from build123d import *

# Parameters (mm, degrees)
SKETCH1_R           = 0.5715
BOSS_EXTRUDE1_DEPTH = 1.5875
CUT_EXTRUDE1_REACH  = 35.788
SKETCH2_W           = 2.901094666
SKETCH2_H           = 2.434307465


with BuildPart() as part:
    # Sketch1 → Boss-Extrude1 (new body)
    with BuildSketch(Plane.XY):
        with BuildLine():
            Line((17.145, 22.225), (-17.145, 22.225))
            ThreePointArc((-17.145, 22.225), (-22.982166479, 19.807166479), (-25.4, 13.97))
            Line((-25.4, 13.97), (-25.4, -13.97))
            ThreePointArc((-25.4, -13.97), (-22.982166479, -19.807166479), (-17.145, -22.225))
            Line((-17.145, -22.225), (17.145, -22.225))
            ThreePointArc((17.145, -22.225), (22.982166479, -19.807166479), (25.4, -13.97))
            Line((25.4, -13.97), (25.4, 13.97))
            ThreePointArc((25.4, 13.97), (22.982166479, 19.807166479), (17.145, 22.225))
        make_face()
        with Locations((-20.759611123, 18.164659732)):
            Circle(SKETCH1_R, mode=Mode.SUBTRACT)
        with Locations(Location((20.759611123, 18.164659732, 0), (0, 0, 180))):
            Circle(SKETCH1_R, mode=Mode.SUBTRACT)
        with BuildLine():
            Line((-17.145, -18.923), (-9.632094666, -18.923))
            Line((-9.632094666, -18.923), (-2.416367182, -12.868285729))
            ThreePointArc((-2.416367182, -12.868285729), (0, -19.5072), (2.416367182, -12.868285729))
            Line((2.416367182, -12.868285729), (9.632094666, -18.923))
            Line((9.632094666, -18.923), (17.145, -18.923))
            ThreePointArc((17.145, -18.923), (20.647299887, -17.472299887), (22.098, -13.97))
            Line((22.098, -13.97), (22.098, 13.97))
            ThreePointArc((22.098, 13.97), (20.647299887, 17.472299887), (17.145, 18.923))
            Line((17.145, 18.923), (-17.145, 18.923))
            ThreePointArc((-17.145, 18.923), (-20.647299887, 17.472299887), (-22.098, 13.97))
            Line((-22.098, 13.97), (-22.098, -13.97))
            ThreePointArc((-22.098, -13.97), (-20.647299887, -17.472299887), (-17.145, -18.923))
        make_face(mode=Mode.SUBTRACT)
    extrude(amount=BOSS_EXTRUDE1_DEPTH)

    # Sketch2 → Cut-Extrude1 (cut, up to next)
    with BuildSketch(Plane.XY.offset(1.5875), mode=Mode.PRIVATE) as cut_extrude1_sk1:
        with Locations((-8.181547333, -17.705846268)):
            Rectangle(SKETCH2_W, SKETCH2_H)
    cut_extrude1_tool1 = extrude(cut_extrude1_sk1.sketch, amount=-CUT_EXTRUDE1_REACH, mode=Mode.PRIVATE) & part.part
    # Sketch2 → Cut-Extrude1 (cut, up to next)
    with BuildSketch(Plane.XY.offset(1.5875), mode=Mode.PRIVATE) as cut_extrude1_sk2:
        with Locations((8.181547333, -17.705846268)):
            Rectangle(SKETCH2_W, SKETCH2_H)
    cut_extrude1_tool2 = extrude(cut_extrude1_sk2.sketch, amount=-CUT_EXTRUDE1_REACH, mode=Mode.PRIVATE) & part.part
    add(cut_extrude1_tool1.solids().sort_by_distance((-8.181547, -17.705846, 1.5875))[0], mode=Mode.SUBTRACT)
    add(cut_extrude1_tool2.solids().sort_by_distance((8.181547, -17.705846, 1.5875))[0], mode=Mode.SUBTRACT)


solid = part.part
CAD build for the part. Positions are in the model's coordinates, mm. A direction names the side the tool comes from. Round coordinates to 2 decimals unless told otherwise and drop trailing zeros. Loops run counter-clockwise (first coordinate to the right, second up) from the corner with the lowest first, then second, coordinate; pieces in that order, holes last. Notation, with made-up numbers: (27.25, -16) - (45.25, -16) arc R21 cw to (45.25, 12) - close; hole circle Ø2 at (77.5, 11.5). An arc over 180 degrees is marked (long way). Put each result on its own line as item: value.
1. Slice it at B-B on x = 11.5. List the corners of the cut face in (y, z) (1 decimal), and give its area (3 significant figures).
Geometry check:
outline: (-22.2, 0) - (-18.9, 0) - (-18.9, 1.6) - (-22.2, 1.6) - close; (18.9, 0) - (22.2, 0) - (22.2, 1.6) - (18.9, 1.6) - close
area: 10.5 mm²
2. Two-plate mould, pull along Y, no slides. Class faces 3 (the cylindrical face through (-22.92, 19.87, 0.78)), 4 (the flat face through (-12, -18.923, 1)), 5 (the flat face through (0, 20, 1.588)): released by +Y, released by -Y, zero draft, split by the parting line, or undercut.
Geometry check:
face 3: released by +Y
face 4: undercut
face 5: zero draft
3. Wall check: line 1 (X direction, y = 4, z = 1.15); line 2 (Y direction, x = 15, z = 0.2) (3 decimals); line 3 (X direction, y = 15.5, z = 1.1). Give the ranges that are in metal, low to high.
Geometry check:
line 1: -25.4 to -22.1, 22.1 to 25.4
line 2: -22.225 to -18.923, 18.923 to 22.225
line 3: -25.26 to -21.86, 21.86 to 25.26
4. Slice it at A-A on y = 12.5. List the corners of the cut face in (x, z), and give its area (3 significant figures).
Geometry check:
outline: (-25.4, 0) - (-22.1, 0) - (-22.1, 1.59) - (-25.4, 1.59) - close; (22.1, 0) - (25.4, 0) - (25.4, 1.59) - (22.1, 1.59) - close
area: 10.5 mm²
5. 3-axis set-ups, long thin cutter, end or side, ignore diameter. For faces 1 (the flat face through (6.731, -18, 1)), 2 (the flat face through (0, 22.225, 1)): which of +Z, -Z, +X, -X, +Y, -Y reach the whole face in a straight line?
Geometry check:
face 1: +Z, -Z
face 2: +Z, -Z, +X, -X, +Y
6. Pin check, flat tips, straight feed: P1, Ø6, axis at x = 16.5, y = 16, coming from the +Z side; P2, Ø0.5, axis at y = -18, z = 1, coming from the +X side; P3, Ø0.5, axis at y = -17.5, z = 1, coming from the -X side. Stop position of each tip, or through.
Geometry check:
P1: z = 1.59
P2: x = 24.48
P3: x = -24.72
